CAD build for the part. Positions are in the model's coordinates, mm. Round coordinates to 2 decimals unless told otherwise and drop trailing zeros. Order: outer loops, then holes, each group sorted by start corner. A loop starts at its lowest first (then second) coordinate and runs counter-clockwise, first axis right, second up. Notation, with made-up numbers: (40, 83.25) -> (60, 83.25) arc R12 cw to (60, 101.25) -> close; hole circle Ø9 at (80, 2). An arc over 180 degrees is marked (long way). Answer as CSV lines item,"result". Start each with the question number.
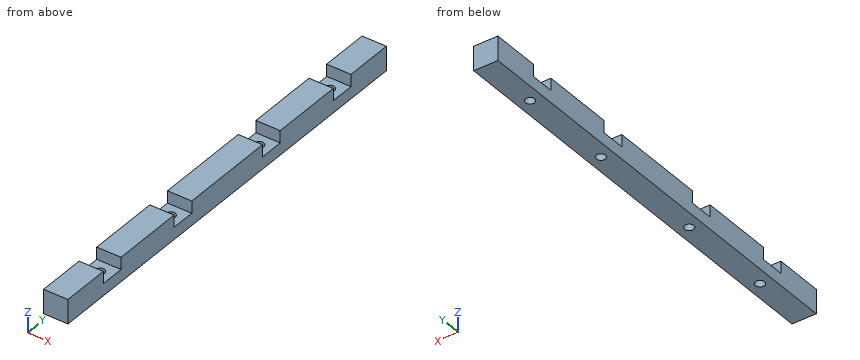
from build123d import *

# Parameters (mm, degrees)
F0_W     = 12.7
F0_H     = 228.6
F1_DEPTH = 12.7
F2_W     = 12.7
F2_H     = 6.35
F3_DEPTH = 12.701
F4_R     = 2.413
F5_DEPTH = 6.351


with BuildPart() as f1:
    # F0 (on Top) → F1 (new body)
    with BuildSketch(Plane.XY):
        with Locations((-6.35, 0)):
            Rectangle(F0_W, F0_H)
    extrude(amount=F1_DEPTH)

    # F2 (on face) → F3 (cut, through all)
    with BuildSketch(Plane.YZ):
        with Locations((82.55, 9.525)):
            Rectangle(F2_W, F2_H)
        with Locations((31.75, 9.525)):
            Rectangle(F2_W, F2_H)
        with Locations((-31.75, 9.525)):
            Rectangle(F2_W, F2_H)
        with Locations((-82.55, 9.525)):
            Rectangle(F2_W, F2_H)
    extrude(amount=-F3_DEPTH, mode=Mode.SUBTRACT)

    # F4 (on face) → F5 (cut, through all)
    with BuildSketch(Plane.XY.offset(6.35)):
        with Locations((-6.35, 82.55)):
            Circle(F4_R)
        with Locations((-6.35, 31.75)):
            Circle(F4_R)
        with Locations((-6.35, -31.75)):
            Circle(F4_R)
        with Locations((-6.35, -82.55)):
            Circle(F4_R)
    extrude(amount=-F5_DEPTH, mode=Mode.SUBTRACT)


solid = f1.part
Item 1: Band-saw the part on C-C, the plane x = -6.35. Count the separate pieces of the cut face and the enclosed holes in it, and give its area (3 significant figures).
Item 2: Probe line 1 (Y direction, x = -7, z = 8.5); line 2 (Y direction, x = -6.35, z = 1.75); line 3 (Z direction, x = -7.75, y = -80.5). List the from-to ranges inside material, lowest first.
Item 3: Band-saw the part on A-A, the plane y = 82.55. Give the cut face in (x, z).
Item 4: Band-saw the part on B-B, the plane z = 3.25. Give the cut face in (x, y), and give its area (3 significant figures).
Item 5: Pin check, flat tips, straight feed: pin 1 (6.5 mm diameter, centred on x = -8.5, y = -84, fed in from +Z); pin 2 (4 mm diameter, centred on x = -6.35, y = 82.55, fed in from -Z). Stop position of each tip, or through.
Values:
1,separate pieces,"5"
1,enclosed holes,"0"
1,area,"2,460 mm²"
2,line 1,"-114.3 to -88.9, -76.2 to -38.1, -25.4 to 25.4, 38.1 to 76.2, 88.9 to 114.3"
2,line 2,"-114.3 to -84.96, -80.14 to -34.16, -29.34 to 29.34, 34.16 to 80.14, 84.96 to 114.3"
2,line 3,"0 to 6.35"
3,outline,"(-12.7, 0) -> (-8.76, 0) -> (-8.76, 6.35) -> (-12.7, 6.35) -> close; (-3.94, 0) -> (0, 0) -> (0, 6.35) -> (-3.94, 6.35) -> close"
4,outline,"(-12.7, -114.3) -> (0, -114.3) -> (0, 114.3) -> (-12.7, 114.3) -> close; hole circle Ø4.83 at (-6.35, -82.55); hole circle Ø4.83 at (-6.35, -31.75); hole circle Ø4.83 at (-6.35, 31.75); hole circle Ø4.83 at (-6.35, 82.55)"
4,area,"2,830 mm²"
5,pin 1,"z = 6.35"
5,pin 2,"through"
